```python
from build123d import *

# Parameters (mm, degrees)
SKETCH3_W           = 20.7
SKETCH3_H           = 24.35
SKETCH3_W_2         = 18.7
SKETCH3_H_2         = 22.35
EXTRUDE_THIN1_DEPTH = 36.95
SKETCH4_W           = 25.5
SKETCH4_H           = 3.65
CUT_EXTRUDE1_DEPTH  = 21.7


with BuildPart() as part:
    # Sketch3 → Extrude-Thin1 (new body)
    with BuildSketch(Plane.XY):
        Rectangle(SKETCH3_W, SKETCH3_H)
        Rectangle(SKETCH3_W_2, SKETCH3_H_2, mode=Mode.SUBTRACT)
    extrude(amount=EXTRUDE_THIN1_DEPTH)

    # Sketch4 → Cut-Extrude1 (cut, through all)
    with BuildSketch(Plane.ZY.offset(10.35)):
        with Locations((24.2, 0)):
            Rectangle(SKETCH4_W, SKETCH4_H)
    extrude(amount=-CUT_EXTRUDE1_DEPTH, mode=Mode.SUBTRACT)


solid = part.part
```
Geometry check sheet. Reference: the model listing, model coordinates, mm. A direction names the side the tool comes from. Round coordinates to 2 decimals unless told otherwise and drop trailing zeros. Loops run counter-clockwise (first coordinate to the right, second up) from the corner with the lowest first, then second, coordinate; pieces in that order, holes last. Notation, with made-up numbers: (62, -6) - (91, -6) arc R15 cw to (91, 11) - close; hole circle Ø6 at (80.25, 2). An arc over 180 degrees is marked (long way). Write item = value, one per line. Start each with the question number.
1. Section check D-D on z = 10. Enter the section's corners in (x, y) (3 decimals).
2. Depth check by flat-ended pin: pin 1 (1.1 mm diameter, centred on x = 9.5, y = -0.5, fed in from +Z). Enter the tip coordinate at first touch or a pass-through.
3. Section check C-C on z = 17.5. Enter the section's corners in (x, y) (3 decimals).
4. Section check A-A on y = 10.5. Enter the section's corners in (x, z), then the cut area to 3 significant figures.
5. Set-up check for faces 5 (the face through (-10, 0, 0)), 6 (the face through (0, -11.175, 18)), 7 (the face through (-10, 1.825, 24)): record each of +Z, -Z, +X, -X, +Y, -Y from which the full face is reachable in a straight line by a thin tool's end or side.
6. Section check B-B on x = -1.75. Enter the section's corners in (y, z) (3 decimals).
7. Mould release check, pull along X, two halves, no side actions. Record for faces 1 (the face through (0, 11.175, 18)), 2 (the face through (9.35, 2, 18)), 3 (the face through (-10.35, -3, 18)), 4 (the face through (0, -12, 36.95)): released by +X, released by -X, zero draft, split by the parting line, or undercut.
8. Thickness scan on line 1 (X direction, y = -1, z = 4.5); line 2 (Y direction, x = -5, z = 31.5) (3 decimals). Record the ranges inside material, lowest first.
Working result:
q1.outline = (-10.35, -12.175) - (10.35, -12.175) - (10.35, 12.175) - (-10.35, 12.175) - close; hole (-9.35, -11.175) - (9.35, -11.175) - (9.35, 11.175) - (-9.35, 11.175) - close
q2.pin_1 = 11.45
q3.outline = (-10.35, -12.175) - (10.35, -12.175) - (10.35, -1.825) - (9.35, -1.825) - (9.35, -11.175) - (-9.35, -11.175) - (-9.35, -1.825) - (-10.35, -1.825) - close; (-10.35, 1.825) - (-9.35, 1.825) - (-9.35, 11.175) - (9.35, 11.175) - (9.35, 1.825) - (10.35, 1.825) - (10.35, 12.175) - (-10.35, 12.175) - close
q4.outline = (-10.35, 0) - (-9.35, 0) - (-9.35, 36.95) - (-10.35, 36.95) - close; (9.35, 0) - (10.35, 0) - (10.35, 36.95) - (9.35, 36.95) - close
q4.area = 73.9 mm^2
q5.face_5 = -Z, +X, -X, +Y, -Y
q5.face_6 = +Z, -Z
q5.face_7 = +Z, +X, -X
q6.outline = (-12.175, 0) - (-11.175, 0) - (-11.175, 36.95) - (-12.175, 36.95) - close; (11.175, 0) - (12.175, 0) - (12.175, 36.95) - (11.175, 36.95) - close
q7.face_1 = undercut
q7.face_2 = undercut
q7.face_3 = released by -X
q7.face_4 = zero draft
q8.line_1 = -10.35 to -9.35, 9.35 to 10.35
q8.line_2 = -12.175 to -11.175, 11.175 to 12.175
